Design review of the part built by this model. Coordinates are the model's own, in mm. A direction names the side the tool comes from. Give positions to 0.01 mm unless a question says otherwise; leave off trailing zeros. Loops run counter-clockwise (first coordinate to the right, second up) from the corner with the lowest first, then second, coordinate; pieces in that order, holes last.
from build123d import *

# Parameters (mm, degrees)
F1_DEPTH       = 4
F3_DEPTH       = 2.83
F6_DEPTH       = 1.171
F7_SIZE        = 0.5
F8_SIZE        = 0.3
F9_R           = 1
F10_DEPTH      = 8
F10_DEPTH_BACK = 8
F11_W          = 9.1
F11_H          = 5.6
F12_DEPTH      = 0.5
F12_DEPTH_BACK = 4.051
F13_R          = 3


with BuildPart() as f1:
    # F0 (on Top) → F1 (new body)
    with BuildSketch(Plane.XY):
        with BuildLine():
            Line((11.9, 11.7878115017), (-11.9, 11.7878115017))
            ThreePointArc((-11.9, 11.7878115017), (-12.2113231748, 11.464993952), (-12.5138921377, 11.1339572285))
            ThreePointArc((-12.5138921377, 11.1339572285), (0.4484386712, -16.7439960212), (11.9, 11.7878115017))
        make_face()
    extrude(amount=F1_DEPTH)

    # F2 (on face) → F3 (cut)
    with BuildSketch(Plane.XY.offset(4)):
        with BuildLine():
            Line((11.8731823496, 10.0878115017), (-11.8731823496, 10.0878115017))
            ThreePointArc((-11.8731823496, 10.0878115017), (0, -15.58), (11.8731823496, 10.0878115017))
        make_face()
    extrude(amount=-F3_DEPTH, mode=Mode.SUBTRACT)

    # F4 (on Front) → F5 (revolve)
    with BuildSketch(Plane.XZ):
        Polygon((4, 1.17), (4.95, 1.17), (4.95, 4.8090074414), (4.7, 4.9), (4.7, 5.05), (4.95, 5.3), (4.95, 6.05), (4, 6.05), align=None)
    revolve(axis=Axis((0, 0, 5.7729503606), (0, 0, 1)))

    # F6 (cut, through all): a face of the model
    f6_faces = [f1.faces().sort_by_distance(p)[0] for p in [
        (0, 0, 1.17),
    ]]
    extrude(f6_faces, amount=-F6_DEPTH, mode=Mode.SUBTRACT)

    # F7
    f7_edges = [f1.edges().sort_by_distance(p)[0] for p in [
        (-4.95, 0, 6.05),
    ]]
    chamfer(f7_edges, length=F7_SIZE)

    # F8
    f8_edges = [f1.edges().sort_by_distance(p)[0] for p in [
        (-4, 0, 6.05),
    ]]
    chamfer(f8_edges, length=F8_SIZE)

    # F9 (on Right) → F10 (join, two sides)
    with BuildSketch(Plane.YZ) as f10_sk:
        with BuildLine():
            Line((13.8378115017, 4), (11.7878115017, 4))
            Line((11.7878115017, 4), (11.7878115017, 0))
            Line((11.7878115017, 0), (13.8378115017, 0))
            ThreePointArc((13.8378115017, 0), (15.8378115017, 2), (13.8378115017, 4))
        make_face()
        with Locations((13.8378115017, 2)):
            Circle(F9_R, mode=Mode.SUBTRACT)
    extrude(amount=F10_DEPTH)
    extrude(f10_sk.sketch, amount=-F10_DEPTH_BACK)

    # F11 (on face) → F12 (cut, two sides)
    with BuildSketch(Plane(origin=(0, 11.7878115017, 0), x_dir=(-1, 0, 0), z_dir=(0, 1, 0))) as f12_sk:
        with Locations((0, 2)):
            Rectangle(F11_W, F11_H)
    extrude(amount=-F12_DEPTH, mode=Mode.SUBTRACT)
    extrude(f12_sk.sketch, amount=F12_DEPTH_BACK, mode=Mode.SUBTRACT)

    # F13
    f13_edges = [f1.edges().sort_by_distance(p)[0] for p in [
        (-11.873182, 10.087812, 2.585),
        (11.873182, 10.087812, 2.585),
    ]]
    fillet(f13_edges, radius=F13_R)


solid = f1.part
Q1. Draft analysis for pull direction X (two halves, no side actions). For faces 1 (the face through (8, 13, 3)), 2 (the face through (-11.78, 9.75, 2.57)), 3 (the face through (-8, 13, 3)), 4 (the face through (-10, 11.788, 2)), state which applies: pulls with the +X half, pulls with the -X half, needs draft (parallel to the pull), parting line crosses it, or undercut.
Results:
face 1: pulls with the +X half
face 2: undercut
face 3: pulls with the -X half
face 4: needs draft
Q2. Insertion check: pin 1 (1.5 mm diameter, centred on y = 8, z = 4.5, fed in from -X); pin 2 (3 mm diameter, centred on y = 13.84, z = 2, fed in from +X); pin 3 (2 mm diameter, centred on x = -10, z = 2, fed in from +Y). Each pin has a flat end and moves straight along its axis. Give the tip position at first contact, or say it passes through.
Results:
pin 1: stops at x = -15.01
pin 2: stops at x = 8
pin 3: stops at y = 11.79
Q3. Take a section at C-C (x = 0). Give the boundary of the cut face in (y, z), plus the area to 3 significant figures.
Results:
outline: (-16.75, 0) - (-4, 0) - (-4, 5.75) - (-4.3, 6.05) - (-4.45, 6.05) - (-4.95, 5.55) - (-4.95, 5.3) - (-4.7, 5.05) - (-4.7, 4.9) - (-4.95, 4.81) - (-4.95, 1.17) - (-15.58, 1.17) - (-15.58, 4) - (-16.75, 4) - close; (4, 0) - (11.29, 0) - (11.29, 4) - (10.09, 4) - (10.09, 1.17) - (4.95, 1.17) - (4.95, 4.81) - (4.7, 4.9) - (4.7, 5.05) - (4.95, 5.3) - (4.95, 5.55) - (4.45, 6.05) - (4.3, 6.05) - (4, 5.75) - close
area: 38.9 mm2
Q4. Wall thickness on line 1 (Y direction, x = 0, z = 3.75); line 2 (Y direction, x = -6.5, z = 1.75); line 3 (Y direction, x = -7, z = 1.5): over which ranges is each line inside the solid? List them lowest first.
Results:
line 1: y = -16.75 to -15.58, -4.95 to -4, 4 to 4.95, 10.09 to 11.29
line 2: y = -15.44 to -14.16, 10.09 to 12.87, 14.81 to 15.82
line 3: y = -15.22 to -13.92, 10.09 to 12.97, 14.7 to 15.77
Q5. Take a section at B-B (z = 2). Give the boundary of the cut face in (x, y), plus the area to 3 significant figures.
Results:
outline: (-11.9, 11.79) arc R16.75 ccw (long way) to (11.9, 11.79) - (8, 11.79) - (8, 12.84) - (4.55, 12.84) - (4.55, 11.29) - (-4.55, 11.29) - (-4.55, 12.84) - (-8, 12.84) - (-8, 11.79) - close; (-8, 14.84) - (-4.55, 14.84) - (-4.55, 15.84) - (-8, 15.84) - close; circle Ø9.9 at (0, 0); (4.55, 14.84) - (8, 14.84) - (8, 15.84) - (4.55, 15.84) - close; hole (-12.87, 8.78) arc R15.58 ccw (long way) to (12.87, 8.78) arc R3 ccw to (10.39, 10.09) - (-10.39, 10.09) arc R3 ccw to start; hole circle Ø8 at (0, 0)
area: 165 mm2
Q6. Take a section at A-A (y = 0). Give the boundary of the cut face in (x, z), plus the area to 3 significant figures.
Results:
outline: (-16.75, 0) - (-4, 0) - (-4, 5.75) - (-4.3, 6.05) - (-4.45, 6.05) - (-4.95, 5.55) - (-4.95, 5.3) - (-4.7, 5.05) - (-4.7, 4.9) - (-4.95, 4.81) - (-4.95, 1.17) - (-15.58, 1.17) - (-15.58, 4) - (-16.75, 4) - close; (4, 0) - (16.75, 0) - (16.75, 4) - (15.58, 4) - (15.58, 1.17) - (4.95, 1.17) - (4.95, 4.81) - (4.7, 4.9) - (4.7, 5.05) - (4.95, 5.3) - (4.95, 5.55) - (4.45, 6.05) - (4.3, 6.05) - (4, 5.75) - close
area: 45.2 mm2
Q7. Tool access review of faces 5 (the face through (0, 11.288, 2)), 6 (the face through (0, 10.088, 3)), 7 (the face through (6.25, 14.79, 2.3)): name each direction out of +Z, -Z, +X, -X, +Y, -Y from which nothing blocks a thin tool from reaching the whole face with its end or side.
Results:
face 5: +Z, -Z, +Y
face 6: +Z
face 7: +X, -X
Q8. Take a section at D-D (y = -12.5). Give the boundary of the cut face in (x, z), plus the area to 3 significant figures.
Results:
outline: (-11.15, 0) - (11.15, 0) - (11.15, 4) - (9.3, 4) - (9.3, 1.17) - (-9.3, 1.17) - (-9.3, 4) - (-11.15, 4) - close
area: 36.6 mm2
